```python
from build123d import *

# Parameters (mm, degrees)
BOSS_EXTRUDE1_DEPTH = 10
CUT_EXTRUDE1_DEPTH  = 5
SKETCH4_R           = 2.6
BOSS_EXTRUDE2_DEPTH = 5
SKETCH5_R           = 2.6
BOSS_EXTRUDE3_DEPTH = 5


with BuildPart() as part:
    # Sketch1 → Boss-Extrude1 (new body)
    with BuildSketch(Plane(origin=(0, 0, 0), x_dir=(1, 0, 0), z_dir=(0, 1, 0))):
        with BuildLine():
            Line((-25.4, 25.4), (25.4, 25.4))
            Line((25.4, 25.4), (25.4, -25.4))
            ThreePointArc((25.4, -25.4), (22.285670886, -32.651726446), (14.882492711, -35.386600333))
            ThreePointArc((14.882492711, -35.386600333), (-20.663123864, -20.663123864), (-35.386600333, 14.882492711))
            ThreePointArc((-35.386600333, 14.882492711), (-32.651726446, 22.285670886), (-25.4, 25.4))
        make_face()
        with BuildLine():
            ThreePointArc((-26.999867981, 15.420553429), (-14.735252362, -14.735252362), (15.420553429, -26.999867981))
            ThreePointArc((15.420553429, -26.999867981), (16.999867981, -25.379446571), (15.379446571, -23.800132019))
            ThreePointArc((15.379446571, -23.800132019), (-12.472510663, -12.472510663), (-23.800132019, 15.379446571))
            ThreePointArc((-23.800132019, 15.379446571), (-25.379446571, 16.999867981), (-26.999867981, 15.420553429))
        make_face(mode=Mode.SUBTRACT)
    extrude(amount=BOSS_EXTRUDE1_DEPTH)

    # Sketch3 → Cut-Extrude1 (cut)
    with BuildSketch(Plane(origin=(0, 10, 0), x_dir=(1, 0, 0), z_dir=(0, 1, 0))):
        with BuildLine():
            ThreePointArc((-30.399999366, 15.402518802), (-17.001804661, -16.989729027), (15.376927769, -30.420552794))
            ThreePointArc((15.376927769, -30.420552794), (20.379445937, -25.423072231), (15.381965374, -20.420554063))
            ThreePointArc((15.381965374, -20.420554063), (-9.927175622, -9.922224237), (-20.400000634, 15.397481198))
            ThreePointArc((-20.400000634, 15.397481198), (-25.397481198, 20.399999366), (-30.399999366, 15.402518802))
        make_face()
    extrude(amount=-CUT_EXTRUDE1_DEPTH, mode=Mode.SUBTRACT)

    # Sketch4 → Boss-Extrude2 (add)
    with BuildSketch(Plane(origin=(25.4, 0, 0), x_dir=(0, 0, -1), z_dir=(1, 0, 0))):
        with BuildLine():
            Line((-15.4, 25.50929881), (-15.4, 0))
            Line((-15.4, 0), (25.4, 0))
            Line((25.4, 0), (25.4, 35.50929881))
            Line((25.4, 35.50929881), (-5.4, 35.50929881))
            ThreePointArc((-5.4, 35.50929881), (-12.471067812, 32.580366621), (-15.4, 25.50929881))
        make_face()
        with Locations((10.4, 25.50929881)):
            Circle(SKETCH4_R, mode=Mode.SUBTRACT)
        with Locations((-5.4, 20)):
            Circle(SKETCH4_R, mode=Mode.SUBTRACT)
    extrude(amount=-BOSS_EXTRUDE2_DEPTH)

    # Sketch5 → Boss-Extrude3 (add)
    with BuildSketch(Plane(origin=(0, 0, -25.4), x_dir=(-1, 0, 0), z_dir=(0, 0, -1))):
        with BuildLine():
            Line((5.4, 35.50929881), (-25.4, 35.50929881))
            Line((-25.4, 35.50929881), (-25.4, 0))
            Line((-25.4, 0), (15.4, 0))
            Line((15.4, 0), (15.4, 25.50929881))
            ThreePointArc((15.4, 25.50929881), (12.471067812, 32.580366621), (5.4, 35.50929881))
        make_face()
        with Locations((5.4, 25.50929881)):
            Circle(SKETCH5_R, mode=Mode.SUBTRACT)
        with Locations((-10.4, 20)):
            Circle(SKETCH5_R, mode=Mode.SUBTRACT)
    extrude(amount=-BOSS_EXTRUDE3_DEPTH)


solid = part.part
```
Can you work these out from the model? Positions are in its coordinate system, mm. A direction names the side the tool comes from. Coordinates: 2 decimals unless noted, no trailing zeros. Loops run counter-clockwise (first coordinate to the right, second up) from the corner with the lowest first, then second, coordinate; pieces in that order, holes last. Notation, with made-up numbers: (59, 44) -> (95, 44) arc R12 cw to (95, 67) -> close; hole circle Ø7 at (-15, 27.5). An arc over 180 degrees is marked (long way). Put each result on its own line as item: value. Start each with the question number.
Q1. For faces 4 (the face through (-12.165, 2.465, 12.776)), 5 (the face through (3, 23, -20.4)), 6 (the face through (-25.3, 7.5, -20.4)), 7 (the face through (6, 18, -25.4)), 8 (the face through (-20.27, 4.93, 21.05)), which set-ups out of +Z, -Z, +X, -X, +Y, -Y let a thin tool reach every point of the face, with its end or its side?
Q2. If I drill on line 1 (Y direction, x = 22.5, z = -10.4); line 2 (Y direction, x = -18, z = 20); line 3 (Z direction, x = 2.5, y = 23), over which ranges is the centre line in solid material (lowest first)? Write a range as [from, to].
Q3. I want a section at A-A (y = 19). Write out the boundary of the cut face in (x, z).
Q4. I want a section at B-B (y = 8). Write out the boundary of the cut face in (x, z), plus the area to 3 significant figures.
Q5. Thinking about a two-plate mould opening in Z: for faces 1 (the face through (23, 18, 15.4)), 2 (the face through (22.935, 22.578, 5.738)), 3 (the face through (10.738, 22.578, -22.935)), which applies, pulls with the +Z half, pulls with the -Z half, needs draft (parallel to the pull), parting line crosses it, or undercut?
Q6. I'm going to push flat-ended pins straight in: P1, Ø4.5, axis at y = 20, z = 5.4, coming from the +X side; P2, Ø7.5, axis at y = 16.5, z = -7, coming from the -X side; P3, Ø5.5, axis at y = 19, z = -23, coming from the -X side; P4, Ø1.5, axis at x = -1.5, z = 15.5, coming from the +Y side. Where does each tip first touch, or does it pass through?
Q7. I want a section at D-D (x = -7). Write out the boundary of the cut face in (y, z).
Q8. I want a section at C-C (z = 22). Write out the boundary of the cut face in (x, y).
Taken from the geometry:
1. face 4: +Y, -Y
1. face 5: +Z, -X, +Y
1. face 6: +Y
1. face 7: -Z, +X, -X, +Y, -Y
1. face 8: +Z, -X, +Y, -Y
2. line 1: y = [0, 22.91], [28.11, 35.51]
2. line 2: y = [0, 10]
2. line 3: z = [-25.4, -20.4]
3. outline: (-15.4, -25.4) -> (8, -25.4) -> (8, -20.4) -> (-15.4, -20.4) -> close; (12.8, -25.4) -> (25.4, -25.4) -> (25.4, 3) -> (20.4, 3) -> (20.4, -20.4) -> (12.8, -20.4) -> close; (20.4, 7.8) -> (25.4, 7.8) -> (25.4, 15.4) -> (20.4, 15.4) -> close
4. outline: (-35.39, -14.88) arc R10 ccw to (-25.4, -25.4) -> (25.4, -25.4) -> (25.4, 25.4) arc R10 ccw to (14.88, 35.39) arc R50.27 ccw to start; hole (-30.4, -15.4) arc R5 ccw to (-20.4, -15.4) arc R35.8 cw to (15.38, 20.42) arc R5 ccw to (15.38, 30.42) arc R45.8 ccw to start
4. area: 2,390 mm2
5. face 1: pulls with the +Z half
5. face 2: undercut
5. face 3: needs draft
6. P1: passes through
6. P2: stops at x = 20.4
6. P3: stops at x = -15.4
6. P4: stops at y = 10
7. outline: (0, -25.4) -> (23.46, -25.4) -> (23.46, -20.4) -> (10, -20.4) -> (10, 12.55) -> (5, 12.55) -> (5, 17.02) -> (0, 17.02) -> close; (0, 20.83) -> (5, 20.83) -> (5, 24.57) -> (10, 24.57) -> (10, 30.37) -> (0, 30.37) -> close; (27.56, -25.4) -> (35.38, -25.4) -> (35.38, -20.4) -> (27.56, -20.4) -> close
8. outline: (-19.27, 0) -> (-4.97, 0) -> (-4.97, 5) -> (-11.07, 5) -> (-11.07, 10) -> (-19.27, 10) -> close; (3.21, 0) -> (25.4, 0) -> (25.4, 10) -> (19.03, 10) -> (19.03, 5) -> (3.21, 5) -> close
